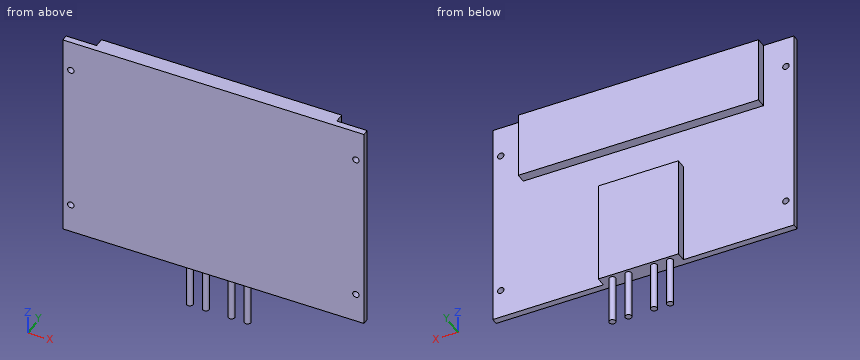
```python
from build123d import *

# Parameters (mm, degrees)
SKETCH_1_W          = 188
SKETCH_1_H          = 132
EXTRUDE_1_DEPTH     = 4
SKETCH_2_W          = 50
SKETCH_2_H          = 65
SKETCH_2_W_2        = 150
SKETCH_2_H_2        = 42
EXTRUDE_2_DEPTH     = 6
SKETCH_3_R          = 2
EXTRUDE_3_DEPTH     = 30
SKETCH_4_R          = 2
CUT_EXTRUDE_1_DEPTH = 10


with BuildPart() as part:
    # 草图1 → 凸台-拉伸1 (new body)
    with BuildSketch(Plane(origin=(0, 0, 0), x_dir=(1, 0, 0), z_dir=(0, 1, 0))):
        with Locations((0, 66)):
            Rectangle(SKETCH_1_W, SKETCH_1_H)
    extrude(amount=EXTRUDE_1_DEPTH)

    # 草图2 → 凸台-拉伸2 (add)
    with BuildSketch(Plane(origin=(0, 4, 0), x_dir=(1, 0, 0), z_dir=(0, 1, 0))):
        with Locations((0, 99.5)):
            Rectangle(SKETCH_2_W, SKETCH_2_H)
        with Locations((0, 21)):
            Rectangle(SKETCH_2_W_2, SKETCH_2_H_2)
    extrude(amount=EXTRUDE_2_DEPTH)

    # 草图3 → 凸台-拉伸3 (add)
    with BuildSketch(Plane(origin=(0, 0, -132), x_dir=(-1, 0, 0), z_dir=(0, 0, -1))):
        with Locations(Location((-18, 6.5, 0), (0, 0, 180))):
            Circle(SKETCH_3_R)
        with Locations(Location((-8, 6.5, 0), (0, 0, 180))):
            Circle(SKETCH_3_R)
        with Locations(Location((8, 6.5, 0), (0, 0, 180))):
            Circle(SKETCH_3_R)
        with Locations(Location((18, 6.5, 0), (0, 0, 180))):
            Circle(SKETCH_3_R)
    extrude(amount=EXTRUDE_3_DEPTH)

    # 草图4 → 切除-拉伸1 (cut)
    with BuildSketch(Plane(origin=(0, 4, 0), x_dir=(1, 0, 0), z_dir=(0, 1, 0))):
        with Locations(Location((89, 113.5, 0), (0, 0, 270))):
            Circle(SKETCH_4_R)
        with Locations(Location((89, 19.5, 0), (0, 0, 270))):
            Circle(SKETCH_4_R)
        with Locations(Location((-89, 19.5, 0), (0, 0, 270))):
            Circle(SKETCH_4_R)
        with Locations(Location((-89, 113.5, 0), (0, 0, 270))):
            Circle(SKETCH_4_R)
    extrude(amount=-CUT_EXTRUDE_1_DEPTH, mode=Mode.SUBTRACT)


solid = part.part
```
For this review, take the finished solid that the model builds, in its own axes (mm). Give positions to 0.01 mm unless a question says otherwise; leave off trailing zeros. Write each loop counter-clockwise with the first axis right and the second up, starting at its lowest first coordinate (ties: lowest second). Pieces come first, ordered by that corner, then holes. Notation, with made-up numbers: M 36,-12.75 L 51,-12.75 A20 ccw 51,20.25 Z; hole C -14,70.5 d3. An arc over 180 degrees is marked long. One line per item, written item: value.
1) Take a section at D-D, the plane x = 18. Write out the cut boundary in (y, z).
Results are:
outline: M 0,-132 L 4.5,-132 L 4.5,-162 L 8.5,-162 L 8.5,-132 L 10,-132 L 10,-67 L 4,-67 L 4,-42 L 10,-42 L 10,0 L 0,0 Z
2) For P1, Ø5, axis at y = 8, z = -94.5, coming from the +X side; P2, Ø3, axis at y = 8, z = -13.5, coming from the +X side; P3, Ø1.8, axis at y = 5.5, z = -108, coming from the -X side; P4, Ø3.5, axis at x = 89, z = -19.5, coming from the +Y side, all flat-tipped, find the tip position at first contact; note any pin that passes through.
Results are:
P1: stops at x = 25
P2: stops at x = 75
P3: stops at x = -25
P4: passes through
3) Take a section at C-C, the plane z = -19.5. Write out the cut boundary in (x, y), then the cut area to 3 significant figures.
Results are:
outline: M -94,0 L -91,0 L -91,4 L -94,4 Z; M -87,0 L 87,0 L 87,4 L 75,4 L 75,10 L -75,10 L -75,4 L -87,4 Z; M 91,0 L 94,0 L 94,4 L 91,4 Z
area: 1,620 mm²
4) For line 1 (X direction, y = 1.1, z = -19.5); line 2 (Z direction, x = -7, y = 5); line 3 (Y direction, x = 0.5, z = -66), list the stretches that pass through material, from the lowest coordinate up. Write a range as from..to.
Results are:
line 1: x = -94..-91, -87..87, 91..94
line 2: z = -162..-67, -42..0
line 3: y = 0..4
5) Take a section at A-A, the plane y = 6.5. Write out the cut boundary in (x, z).
Results are:
outline: M -75,-42 L 75,-42 L 75,0 L -75,0 Z; M -25,-132 L -20,-132 L -20,-162 L -16,-162 L -16,-132 L -10,-132 L -10,-162 L -6,-162 L -6,-132 L 6,-132 L 6,-162 L 10,-162 L 10,-132 L 16,-132 L 16,-162 L 20,-162 L 20,-132 L 25,-132 L 25,-67 L -25,-67 Z
6) Take a section at B-B, the plane x = 89. Write out the cut boundary in (y, z), then the cut area to 3 significant figures.
Results are:
outline: M 0,-132 L 4,-132 L 4,-115.5 L 0,-115.5 Z; M 0,-111.5 L 4,-111.5 L 4,-21.5 L 0,-21.5 Z; M 0,-17.5 L 4,-17.5 L 4,0 L 0,0 Z
area: 496 mm²
